```python
from build123d import *

# Parameters (mm, degrees)
SKETCH1_W            = 14.28
SKETCH1_H            = 14.28
BOSS_EXTRUDE1_DEPTH  = 1.5
SKETCH3_W            = 1.5
SKETCH3_H            = 1.5
BOSS_EXTRUDE3_DEPTH  = 12
LPATTERN2_COUNT      = 5
LPATTERN2_PITCH      = 3
LPATTERN2_COUNT_DIR2 = 5
LPATTERN2_PITCH_DIR2 = 3


with BuildPart() as part:
    # Sketch1 → Boss-Extrude1 (new body)
    with BuildSketch(Plane(origin=(0, 0, 0), x_dir=(1, 0, 0), z_dir=(0, 1, 0))):
        Rectangle(SKETCH1_W, SKETCH1_H)
    extrude(amount=BOSS_EXTRUDE1_DEPTH)

    # Sketch3 → Boss-Extrude3 (add)
    with BuildSketch(Plane(origin=(0, 1.5, 0), x_dir=(1, 0, 0), z_dir=(0, 1, 0))):
        with Locations((-6.39, 6.39)):
            Rectangle(SKETCH3_W, SKETCH3_H)
    boss_extrude3 = extrude(amount=BOSS_EXTRUDE3_DEPTH)

    # LPattern2: Boss-Extrude3 5 × 5
    with Locations(*[(i * LPATTERN2_PITCH, 0, j * LPATTERN2_PITCH_DIR2) for i in range(LPATTERN2_COUNT) for j in range(LPATTERN2_COUNT_DIR2) if (i, j) != (0, 0)]):
        add(boss_extrude3)


solid = part.part
```
Could you check a few things on this model? Use its own coordinates, in mm. A direction names the side the tool comes from. Coordinates: 2 decimals unless noted, no trailing zeros. Loops run counter-clockwise (first coordinate to the right, second up) from the corner with the lowest first, then second, coordinate; pieces in that order, holes last. Notation, with made-up numbers: M 23,-35.75 L 28,-35.75 A6 cw 28,-30.75 Z; hole C -33,31.25 d7. An arc over 180 degrees is marked long. Put each result on its own line as item: value. Start each with the question number.
(1) Suppose I cut it at D-D on x = 4.25. Please give me the cut outline in (y, z), then the cut area to 3 significant figures.
(2) Suppose I cut it at C-C on x = 0. Please give me the cut outline in (y, z), then the cut area to 3 significant figures.
(3) Will these pins go through, and if not, where does the flat tip stop? P1, Ø3, axis at x = 3.5, y = 6, coming from the +Z side; P2, Ø0.8, axis at y = 7.5, z = -6.5, coming from the +X side.
(4) Suppose I cut it at B-B on z = -0.5. Please give me the cut outline in (x, y).
(5) I need wall thicknesses on line 1 (Z direction, x = -6.25, y = 11.75); line 2 (Y direction, x = 1.25, z = -2). Which ranges of each line are inside material? Lowest first, please. Write a range as from..to.
(6) Suppose I cut it at A-A on y = 8.25. Count the separate pieces of the cut face and the enclosed holes in it, then the cut area to 4 significant figures.
(7) For faces 1 (the face through (3, 7, 6.36)), 2 (the face through (6, 13.5, 0)), 3 (the face through (0, 7, 4.86)), 4 (the face through (-4.14, 7, -3)), which set-ups out of +Z, -Z, +X, -X, +Y, -Y let a thin tool reach every point of the face, with its end or its side?
Solutions:
1. outline: M 0,-7.14 L 1.5,-7.14 L 1.5,7.14 L 0,7.14 Z
1. area: 21.4 mm2
2. outline: M 0,-7.14 L 13.5,-7.14 L 13.5,-5.64 L 1.5,-5.64 L 1.5,-4.14 L 13.5,-4.14 L 13.5,-2.64 L 1.5,-2.64 L 1.5,-1.14 L 13.5,-1.14 L 13.5,0.36 L 1.5,0.36 L 1.5,1.86 L 13.5,1.86 L 13.5,3.36 L 1.5,3.36 L 1.5,4.86 L 13.5,4.86 L 13.5,6.36 L 1.5,6.36 L 1.5,7.14 L 0,7.14 Z
2. area: 111 mm2
3. P1: stops at z = 6.36
3. P2: stops at x = 6.36
4. outline: M -7.14,0 L 7.14,0 L 7.14,1.5 L 6.36,1.5 L 6.36,13.5 L 4.86,13.5 L 4.86,1.5 L 3.36,1.5 L 3.36,13.5 L 1.86,13.5 L 1.86,1.5 L 0.36,1.5 L 0.36,13.5 L -1.14,13.5 L -1.14,1.5 L -2.64,1.5 L -2.64,13.5 L -4.14,13.5 L -4.14,1.5 L -5.64,1.5 L -5.64,13.5 L -7.14,13.5 Z
5. line 1: z = -7.14..-5.64, -4.14..-2.64, -1.14..0.36, 1.86..3.36, 4.86..6.36
5. line 2: y = 0..1.5
6. separate pieces: 25
6. enclosed holes: 0
6. area: 56.25 mm2
7. face 1: +Z, +X, -X, +Y
7. face 2: +Z, -Z, +X, -X, +Y
7. face 3: +X, -X, +Y
7. face 4: +Z, -Z, +Y
